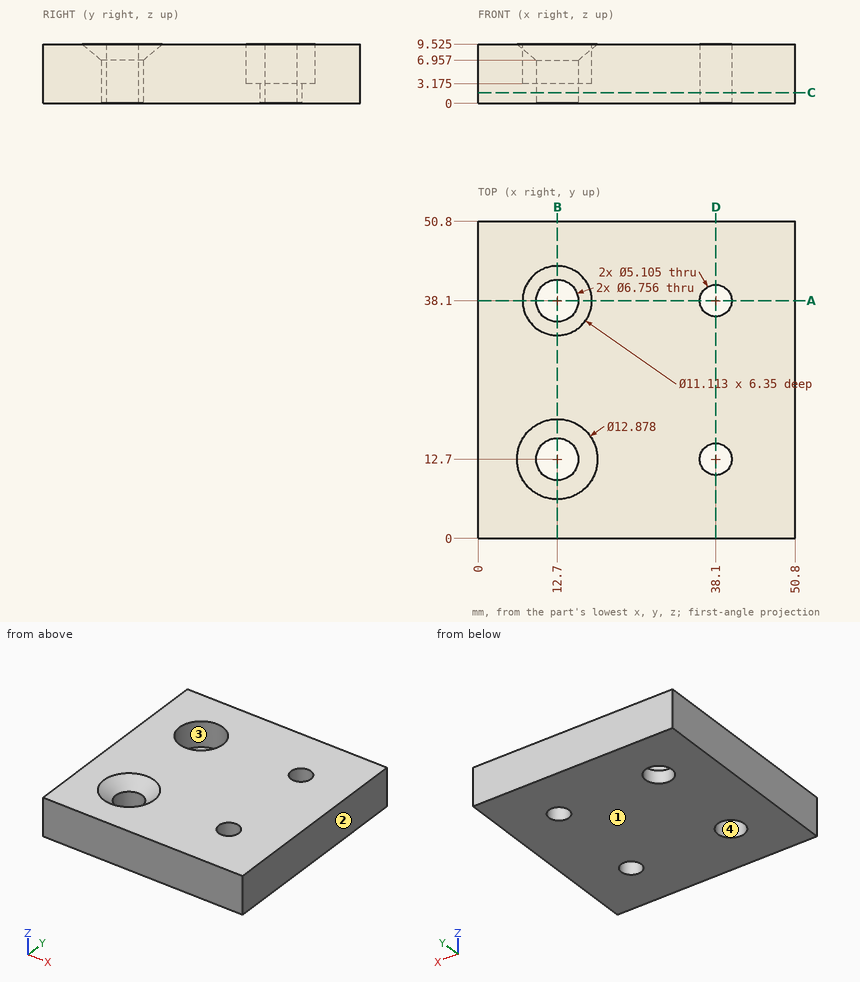
Geometry check sheet. Reference: drawing and pictorial views, mm from the part's lowest x, y, z. Give positions to 0.01 mm unless a question says otherwise; leave off trailing zeros. Order: outer loops, then holes, each group sorted by start corner. A loop starts at its lowest first (then second) coordinate and runs counter-clockwise, first axis right, second up. Notation, with made-up numbers: (50.5, 72.5) - (78.5, 72.5) arc R11 cw to (78.5, 80.5) - close; hole circle Ø9 at (34.5, -14). An arc over 180 degrees is marked (long way). Answer as CSV lines item,"result". Start each with the question number.
Item 1: Section check A-A, the plane y = 38.1. Record the boundary of the cut face in (x, z) (1 decimal), plus the area to 3 significant figures.
Item 2: Section check C-C, the plane z = 1.75. Record the boundary of the cut face in (x, y) (1 decimal).
Item 3: Mould release check, pull along X, two halves, no side actions. Record for the marked faces 1, 2, 3 and 4: released by +X, released by -X, zero draft, split by the parting line, or undercut.
Item 4: Material ranges on L1, parallel to Y at x = 12.7, z = 5.5; L2, parallel to Y at x = 12.7, z = 1.75; L3, parallel to X at y = 11, z = 6 (1 decimal), recorded low to high.
Item 5: Gauge pin test, flat ends, axial feed: pin 1 (11 mm diameter, centred on x = 12.7, y = 12.7, fed in from +Z); pin 2 (4 mm diameter, centred on x = 12.7, y = 38.1, fed in from -Z). Record the tip position at first contact, or that the pin passes through.
Item 6: Section check D-D, the plane x = 38.1. Record the boundary of the cut face in (y, z) (1 decimal).
Item 7: Section check B-B, the plane x = 12.7. Record the boundary of the cut face in (y, z) (1 decimal).
Filled in:
1,outline,"(0, 0) - (9.3, 0) - (9.3, 3.2) - (7.1, 3.2) - (7.1, 9.5) - (0, 9.5) - close; (16.1, 0) - (35.5, 0) - (35.5, 9.5) - (18.3, 9.5) - (18.3, 3.2) - (16.1, 3.2) - close; (40.7, 0) - (50.8, 0) - (50.8, 9.5) - (40.7, 9.5) - close"
1,area,"343 mm^2"
2,outline,"(0, 0) - (50.8, 0) - (50.8, 50.8) - (0, 50.8) - close; hole circle Ø6.8 at (12.7, 12.7); hole circle Ø6.8 at (12.7, 38.1); hole circle Ø5.1 at (38.1, 12.7); hole circle Ø5.1 at (38.1, 38.1)"
3,face 1,"zero draft"
3,face 2,"released by +X"
3,face 3,"undercut"
3,face 4,"undercut"
4,L1,"0 to 9.32, 16.08 to 32.54, 43.66 to 50.8"
4,L2,"0 to 9.32, 16.08 to 34.72, 41.48 to 50.8"
4,L3,"0 to 9.8, 15.6 to 36.2, 40 to 50.8"
5,pin 1,"z = 8.74"
5,pin 2,"through"
6,outline,"(0, 0) - (10.1, 0) - (10.1, 9.5) - (0, 9.5) - close; (15.3, 0) - (35.5, 0) - (35.5, 9.5) - (15.3, 9.5) - close; (40.7, 0) - (50.8, 0) - (50.8, 9.5) - (40.7, 9.5) - close"
7,outline,"(0, 0) - (9.3, 0) - (9.3, 7) - (6.3, 9.5) - (0, 9.5) - close; (16.1, 0) - (34.7, 0) - (34.7, 3.2) - (32.5, 3.2) - (32.5, 9.5) - (19.1, 9.5) - (16.1, 7) - close; (41.5, 0) - (50.8, 0) - (50.8, 9.5) - (43.7, 9.5) - (43.7, 3.2) - (41.5, 3.2) - close"
